from build123d import *

# Parameters (mm, degrees)
SKETCH1_R           = 9
BOSS_EXTRUDE1_DEPTH = 10
FILLET11_R          = 2.5


with BuildPart() as part:
    # Sketch1 → Boss-Extrude1 (new body)
    with BuildSketch(Plane(origin=(0, 0, 0), x_dir=(1, 0, 0), z_dir=(0, 1, 0))):
        with BuildLine():
            Line((25, 0), (5, 113.425636392))
            Line((5, 113.425636392), (-5, 113.425636392))
            Line((-5, 113.425636392), (-25, 0))
            ThreePointArc((-25, 0), (0, -25), (25, 0))
        make_face()
        with Locations(Location((0, 0, 0), (0, 0, 270))):
            Circle(SKETCH1_R, mode=Mode.SUBTRACT)
    extrude(amount=BOSS_EXTRUDE1_DEPTH)

    # Sketch4 → Loft2 section 0
    with BuildSketch(Plane(origin=(0, 0, -113.425636392), x_dir=(-1, 0, 0), z_dir=(0, 0, -1)), mode=Mode.PRIVATE) as loft2_s0:
        with BuildLine():
            Line((-5, 10), (5, 10))
            Line((5, 10), (5, 0))
            Line((5, 0), (-5, 0))
            Line((-5, 0), (-5, 10))
        make_face()
    loft([loft2_s0.sketch, Vertex(0, 5, -143.425636392)])

    # Fillet11
    fillet11_edges = [part.edges().sort_by_distance(p)[0] for p in [
        (15, 0, -56.712818196),
        (15, 10, -56.712818196),
        (-15, 0, -56.712818196),
        (-15, 10, -56.712818196),
    ]]
    fillet(fillet11_edges, radius=FILLET11_R)


solid = part.part
Here's how the part is built. I have some questions about the finished solid (model axes, mm). Give positions to 0.01 mm unless a question says otherwise; leave off trailing zeros. Answer as a JSON object with one key per item and string values. Group by question number.
1) We'd pull the mould along Z, two halves only. Please class faces 1 (the flat face through (0, 10, -30)), 2 (the flat face through (-3.02, 5.04, -125.3)), 3 (the cylindrical face through (2.703, 4.93, 8.584)): pulls with the +Z half, pulls with the -Z half, needs draft (parallel to the pull), parting line crosses it, or undercut.
2) Please list where these lines run through material, in increasing order: L1, parallel to X at y = 7.75, z = 0; L2, parallel to X at y = 8, z = -75; L3, parallel to X at y = 1.75, z = -96.5. Write a range as [from, to].
3) I'm going to push flat-ended pins straight in: pin 1 Ø1 at (y, z) = (2.5, 5.5) entering from +X; pin 2 Ø2 at (x, y) = (7, 3) entering from +Z; pin 3 Ø4 at (x, z) = (15.5, -59.5) entering from +Y. Where does each tip first touch, or does it pass through?
Results found:
{
 "1": {"face 1": "needs draft", "face 2": "pulls with the -Z half", "face 3": "undercut"},
 "2": {"L1": "[-24.99, -9], [9, 24.99]", "L2": "[-11.72, 11.72]", "L3": "[-7.87, 7.87]"},
 "3": {"pin 1": "x = 24.49", "pin 2": "z = 24.27", "pin 3": "y = 9.52"}
}
